Can you work these out from the model? Positions are in its coordinate system, mm. Face numbers are marked on the shaded views. A direction names the side the tool comes from. Give positions to 0.01 mm unless a question says otherwise; leave off trailing zeros. Loops run counter-clockwise (first coordinate to the right, second up) from the corner with the lowest first, then second, coordinate; pieces in that order, holes last. Notation, with made-up numbers: M -7,36.25 L 47,36.25 A34 cw 47,70.25 Z; hole C -37.5,82.25 d7. An arc over 180 degrees is marked long. One line per item, written item: value. Start each with the question number.
from build123d import *

# Parameters (mm, degrees)
BOSS_EXTRUDE2_DEPTH  = 15
BOSS_EXTRUDE3_DEPTH  = 5
SKETCH7_R            = 3.75
BOSS_EXTRUDE9_DEPTH  = 10
SKETCH9_R            = 1.375
CUT_EXTRUDE5_DEPTH   = 21
CUT_EXTRUDE9_REACH   = 131.287
SKETCH14_R           = 8
CUT_EXTRUDE11_REACH  = 105.053
SKETCH16_R           = 8
CUT_EXTRUDE12_REACH  = 131.287
SKETCH17_R           = 8
CUT_EXTRUDE13_REACH  = 121.393
SKETCH19_R           = 8
CUT_EXTRUDE14_REACH  = 121.393
SKETCH20_R           = 8
BOSS_EXTRUDE11_DEPTH = 55
FILLET1_R            = 10
SKETCH25_R           = 4
SKETCH25_R_2         = 1.4
BOSS_EXTRUDE12_DEPTH = 5
SKETCH24_R           = 3.75
CUT_EXTRUDE15_DEPTH  = 65
CUT_EXTRUDE17_REACH  = 105.053
SKETCH26_W           = 58.5
SKETCH26_H           = 18
BOSS_EXTRUDE13_REACH = 77
SKETCH27_R           = 4
SKETCH28_R           = 1.375
CUT_EXTRUDE18_DEPTH  = 25
SKETCH30_R           = 8
CUT_EXTRUDE19_DEPTH  = 122.75
SKETCH31_R           = 8
CUT_EXTRUDE20_DEPTH  = 1.5
SKETCH33_W           = 27
SKETCH33_H           = 4
CUT_EXTRUDE21_DEPTH  = 40
SKETCH35_R           = 1.25
SKETCH35_W           = 9
SKETCH35_H           = 9
CUT_EXTRUDE22_DEPTH  = 7.75


with BuildPart() as part:
    # Sketch1 → Boss-Extrude2 (new body)
    with BuildSketch(Plane(origin=(0, 0, 0), x_dir=(1, 0, 0), z_dir=(0, 1, 0))):
        Polygon((-43.178681761, 29.873916914), (-17.5, 45.604089113), (-17.5, 57.803420417), (17.5, 57.803420417), (17.5, 45.604089113), (43.178681761, 29.873916914), (59, 2.406681305), (59, -41.5), (-59, -41.5), (-59, 2.406681305), align=None)
        Polygon((39.481402229, 26.275231503), (12.5, 42.803420417), (12.5, 52.803420417), (-12.5, 52.803420417), (-12.5, 42.803420417), (-39.481402229, 26.275231503), (-54, 1.069636136), (-54, -38.5), (54, -38.5), (54, 1.069636136), align=None, mode=Mode.SUBTRACT)
    extrude(amount=BOSS_EXTRUDE2_DEPTH)

    # Sketch2 → Boss-Extrude3 (add)
    with BuildSketch(Plane.XZ):
        Polygon((-59, -2.406681305), (-59, 41.5), (59, 41.5), (59, -2.406681305), (43.178681761, -29.873916914), (43.178681761, -57.803420417), (-43.178681761, -57.803420417), (-43.178681761, -29.873916914), align=None)
    extrude(amount=BOSS_EXTRUDE3_DEPTH)

    # Sketch7 → Boss-Extrude9 (add)
    with BuildSketch(Plane(origin=(0, 15, 0), x_dir=(1, 0, 0), z_dir=(0, 1, 0))):
        with Locations((-59, -41.5)):
            Circle(SKETCH7_R)
        with Locations((-59, 2.406681305)):
            Circle(SKETCH7_R)
        with Locations((-43.178681761, 29.873916914)):
            Circle(SKETCH7_R)
        with Locations((-17.5, 57.803420417)):
            Circle(SKETCH7_R)
        with Locations((17.5, 57.803420417)):
            Circle(SKETCH7_R)
        with Locations((43.178681761, 29.873916914)):
            Circle(SKETCH7_R)
        with Locations((59, 2.406681305)):
            Circle(SKETCH7_R)
        with Locations((59, -41.5)):
            Circle(SKETCH7_R)
    extrude(amount=-BOSS_EXTRUDE9_DEPTH)

    # Sketch9 → Cut-Extrude5 (cut, through all)
    with BuildSketch(Plane(origin=(0, 15, 0), x_dir=(1, 0, 0), z_dir=(0, 1, 0))):
        with Locations((-59, -41.5)):
            Circle(SKETCH9_R)
        with Locations((-59, 2.406681305)):
            Circle(SKETCH9_R)
        with Locations((-17.5, 57.803420417)):
            Circle(SKETCH9_R)
        with Locations((43.178681761, 29.873916914)):
            Circle(SKETCH9_R)
        with Locations((17.5, 57.803420417)):
            Circle(SKETCH9_R)
        with Locations((-43.178681761, 29.873916914)):
            Circle(SKETCH9_R)
        with Locations((59, 2.406681305)):
            Circle(SKETCH9_R)
        with Locations((59, -41.5)):
            Circle(SKETCH9_R)
    extrude(amount=-CUT_EXTRUDE5_DEPTH, mode=Mode.SUBTRACT)

    # Sketch14 → Cut-Extrude9 (cut, up to next)
    with BuildSketch(Plane(origin=(-45.342387005, 0, -26.117529435), x_dir=(-0.499126718, 0, 0.866529006), z_dir=(-0.866529006, 0, -0.499126718)), mode=Mode.PRIVATE) as cut_extrude9_sk1:
        with Locations((11.514017709, 15)):
            Circle(SKETCH14_R)
    cut_extrude9_tool1 = extrude(cut_extrude9_sk1.sketch, amount=-CUT_EXTRUDE9_REACH, mode=Mode.PRIVATE) & part.part
    add(cut_extrude9_tool1.solids().sort_by_distance((-51.089341, 15, -16.140299))[0], mode=Mode.SUBTRACT)

    # Sketch16 → Cut-Extrude11 (cut, up to next)
    with BuildSketch(Plane(origin=(0, 0, -57.803420417), x_dir=(-1, 0, 0), z_dir=(0, 0, -1)), mode=Mode.PRIVATE) as cut_extrude11_sk1:
        with Locations((0, 15)):
            Circle(SKETCH16_R)
    cut_extrude11_tool1 = extrude(cut_extrude11_sk1.sketch, amount=-CUT_EXTRUDE11_REACH, mode=Mode.PRIVATE) & part.part
    add(cut_extrude11_tool1.solids().sort_by_distance((0, 15, -57.80342))[0], mode=Mode.SUBTRACT)

    # Sketch17 → Cut-Extrude12 (cut, up to next)
    with BuildSketch(Plane(origin=(45.342387005, 0, -26.117529435), x_dir=(-0.499126718, 0, -0.866529006), z_dir=(0.866529006, 0, -0.499126718)), mode=Mode.PRIVATE) as cut_extrude12_sk1:
        with Locations((-11.514017709, 15)):
            Circle(SKETCH17_R)
    cut_extrude12_tool1 = extrude(cut_extrude12_sk1.sketch, amount=-CUT_EXTRUDE12_REACH, mode=Mode.PRIVATE) & part.part
    add(cut_extrude12_tool1.solids().sort_by_distance((51.089341, 15, -16.140299))[0], mode=Mode.SUBTRACT)

    # Sketch19 → Cut-Extrude13 (cut, up to next)
    with BuildSketch(Plane(origin=(-25.088449392, 0, -40.955578852), x_dir=(-0.852725133, 0, 0.522359882), z_dir=(-0.522359882, 0, -0.852725133)), mode=Mode.PRIVATE) as cut_extrude13_sk1:
        with Locations((4.464611438, 15)):
            Circle(SKETCH19_R)
    cut_extrude13_tool1 = extrude(cut_extrude13_sk1.sketch, amount=-CUT_EXTRUDE13_REACH, mode=Mode.PRIVATE) & part.part
    add(cut_extrude13_tool1.solids().sort_by_distance((-28.895536, 15, -38.623445))[0], mode=Mode.SUBTRACT)

    # Sketch20 → Cut-Extrude14 (cut, up to next)
    with BuildSketch(Plane(origin=(25.088449392, 0, -40.955578852), x_dir=(-0.852725133, 0, -0.522359882), z_dir=(0.522359882, 0, -0.852725133)), mode=Mode.PRIVATE) as cut_extrude14_sk1:
        with Locations((-4.464611438, 15)):
            Circle(SKETCH20_R)
    cut_extrude14_tool1 = extrude(cut_extrude14_sk1.sketch, amount=-CUT_EXTRUDE14_REACH, mode=Mode.PRIVATE) & part.part
    add(cut_extrude14_tool1.solids().sort_by_distance((28.895536, 15, -38.623445))[0], mode=Mode.SUBTRACT)

    # Sketch21 → Boss-Extrude11 (add)
    with BuildSketch(Plane.XZ.offset(5)):
        Polygon((59, 41.5), (59, -2.406681305), (43.178681761, -29.873916914), (43.178681761, -57.803420417), (-43.178681761, -57.803420417), (-43.178681761, -29.873916914), (-59, -2.406681305), (-59, 41.5), align=None)
        Polygon((54, 38.5), (-54, 38.5), (-54, -1.069636136), (-38.178681761, -28.536871745), (-38.178681761, -52.803420417), (38.178681761, -52.803420417), (38.178681761, -28.536871745), (54, -1.069636136), align=None, mode=Mode.SUBTRACT)
    extrude(amount=BOSS_EXTRUDE11_DEPTH)

    # Fillet1
    fillet1_edges = [part.edges().sort_by_distance(p)[0] for p in [
        (43.178681761, -30, -57.803420417),
        (-43.178681761, -30, -57.803420417),
    ]]
    fillet(fillet1_edges, radius=FILLET1_R)

    # Sketch25 → Boss-Extrude12 (add)
    with BuildSketch(Plane(origin=(0, -5, 0), x_dir=(-1, 0, 0), z_dir=(0, -1, 0))):
        with Locations((-24.5, 40.5)):
            Circle(SKETCH25_R)
        with Locations((-24.5, 40.5)):
            Circle(SKETCH25_R_2, mode=Mode.SUBTRACT)
        with Locations((24.5, 40.5)):
            Circle(SKETCH25_R)
        with Locations((24.5, 40.5)):
            Circle(SKETCH25_R_2, mode=Mode.SUBTRACT)
        with Locations((24.5, -17.5)):
            Circle(SKETCH25_R)
        with Locations((24.5, -17.5)):
            Circle(SKETCH25_R_2, mode=Mode.SUBTRACT)
        with Locations((-24.5, -17.5)):
            Circle(SKETCH25_R)
        with Locations((-24.5, -17.5)):
            Circle(SKETCH25_R_2, mode=Mode.SUBTRACT)
    extrude(amount=BOSS_EXTRUDE12_DEPTH)

    # Sketch24 → Cut-Extrude15 (cut)
    with BuildSketch(Plane.XZ.offset(60)):
        with Locations((59, 41.5)):
            Circle(SKETCH24_R)
        with Locations((59, -2.406681305)):
            Circle(SKETCH24_R)
        with Locations((43.178681761, -29.873916914)):
            Circle(SKETCH24_R)
        with Locations((17.5, -57.803420417)):
            Circle(SKETCH24_R)
        with Locations((-17.5, -57.803420417)):
            Circle(SKETCH24_R)
        with Locations((-43.178681761, -29.873916914)):
            Circle(SKETCH24_R)
        with Locations((-59, -2.406681305)):
            Circle(SKETCH24_R)
        with Locations((-59, 41.5)):
            Circle(SKETCH24_R)
    extrude(amount=-CUT_EXTRUDE15_DEPTH, mode=Mode.SUBTRACT)

    # Sketch26 → Cut-Extrude17 (cut, up to next)
    with BuildSketch(Plane.XY.offset(41.5), mode=Mode.PRIVATE) as cut_extrude17_sk1:
        with Locations((0, -19)):
            Rectangle(SKETCH26_W, SKETCH26_H)
    cut_extrude17_tool1 = extrude(cut_extrude17_sk1.sketch, amount=-CUT_EXTRUDE17_REACH, mode=Mode.PRIVATE) & part.part
    add(cut_extrude17_tool1.solids().sort_by_distance((0, -19, 41.5))[0], mode=Mode.SUBTRACT)

    # Sketch27 → Boss-Extrude13 (add, up to next)
    with BuildSketch(Plane(origin=(0, -60, 0), x_dir=(-1, 0, 0), z_dir=(0, -1, 0)), mode=Mode.PRIVATE) as boss_extrude13_sk1:
        with Locations((-51.25, -35.75)):
            Circle(SKETCH27_R)
    boss_extrude13_tool1 = extrude(boss_extrude13_sk1.sketch, amount=-BOSS_EXTRUDE13_REACH, mode=Mode.PRIVATE) - part.part
    add(boss_extrude13_tool1.solids().sort_by_distance((51.25, -60, 35.75))[0])
    # Sketch27 → Boss-Extrude13 (add, up to next)
    with BuildSketch(Plane(origin=(0, -60, 0), x_dir=(-1, 0, 0), z_dir=(0, -1, 0)), mode=Mode.PRIVATE) as boss_extrude13_sk2:
        with Locations((-35.428681761, 50.053420417)):
            Circle(SKETCH27_R)
    boss_extrude13_tool2 = extrude(boss_extrude13_sk2.sketch, amount=-BOSS_EXTRUDE13_REACH, mode=Mode.PRIVATE) - part.part
    add(boss_extrude13_tool2.solids().sort_by_distance((35.428682, -60, -50.05342))[0])
    # Sketch27 → Boss-Extrude13 (add, up to next)
    with BuildSketch(Plane(origin=(0, -60, 0), x_dir=(-1, 0, 0), z_dir=(0, -1, 0)), mode=Mode.PRIVATE) as boss_extrude13_sk3:
        with Locations((35.428681761, 50.053420417)):
            Circle(SKETCH27_R)
    boss_extrude13_tool3 = extrude(boss_extrude13_sk3.sketch, amount=-BOSS_EXTRUDE13_REACH, mode=Mode.PRIVATE) - part.part
    add(boss_extrude13_tool3.solids().sort_by_distance((-35.428682, -60, -50.05342))[0])
    # Sketch27 → Boss-Extrude13 (add, up to next)
    with BuildSketch(Plane(origin=(0, -60, 0), x_dir=(-1, 0, 0), z_dir=(0, -1, 0)), mode=Mode.PRIVATE) as boss_extrude13_sk4:
        with Locations((51.25, -35.75)):
            Circle(SKETCH27_R)
    boss_extrude13_tool4 = extrude(boss_extrude13_sk4.sketch, amount=-BOSS_EXTRUDE13_REACH, mode=Mode.PRIVATE) - part.part
    add(boss_extrude13_tool4.solids().sort_by_distance((-51.25, -60, 35.75))[0])

    # Sketch28 → Cut-Extrude18 (cut)
    with BuildSketch(Plane(origin=(0, -60, 0), x_dir=(-1, 0, 0), z_dir=(0, -1, 0))):
        with Locations((-51.25, -35.75)):
            Circle(SKETCH28_R)
        with Locations((-35.428681761, 50.053420417)):
            Circle(SKETCH28_R)
        with Locations((35.428681761, 50.053420417)):
            Circle(SKETCH28_R)
        with Locations((51.25, -35.75)):
            Circle(SKETCH28_R)
    extrude(amount=-CUT_EXTRUDE18_DEPTH, mode=Mode.SUBTRACT)

    # Sketch30 → Cut-Extrude19 (cut, through all)
    with BuildSketch(Plane.ZY.offset(59)):
        with Locations((13.34, 15)):
            Circle(SKETCH30_R)
    extrude(amount=-CUT_EXTRUDE19_DEPTH, mode=Mode.SUBTRACT)

    # Sketch31 → Cut-Extrude20 (cut)
    with BuildSketch(Plane(origin=(0, 0, 38.5), x_dir=(-1, 0, 0), z_dir=(0, 0, -1))):
        with Locations((-38, 15)):
            Circle(SKETCH31_R)
    extrude(amount=-CUT_EXTRUDE20_DEPTH, mode=Mode.SUBTRACT)

    # Sketch33 → Cut-Extrude21 (cut)
    with BuildSketch(Plane.XZ.offset(60)):
        with Locations((0, -52.803420417)):
            Rectangle(SKETCH33_W, SKETCH33_H)
    extrude(amount=-CUT_EXTRUDE21_DEPTH, mode=Mode.SUBTRACT)

    # Sketch35 → Cut-Extrude22 (cut, through all)
    with BuildSketch(Plane.XY.offset(-54.803420417)):
        with Locations((10.5, -35.5)):
            Circle(SKETCH35_R)
        with Locations((-10.5, -35.5)):
            Circle(SKETCH35_R)
        with Locations((-10.5, -23)):
            Circle(SKETCH35_R)
        with Locations((10.5, -23)):
            Circle(SKETCH35_R)
        with Locations((0, -35.5)):
            Rectangle(SKETCH35_W, SKETCH35_H)
    extrude(amount=-CUT_EXTRUDE22_DEPTH, mode=Mode.SUBTRACT)


solid = part.part
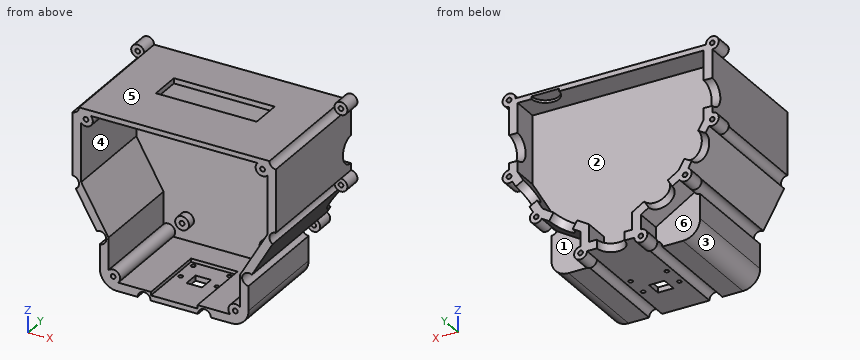
Q1. If we mould it in two halves opening along X, with no side actions, what happens to the marked faces 1, 2 and 3? For each: released by +X, released by -X, zero draft, split by the parting line, or undercut.
Q2. For P1, Ø1.5, axis at y = -33.5, z = -56, coming from the +X side; P2, Ø12, axis at x = 29.5, z = -2.5, coming from the +Y side; P3, Ø14, axis at x = 5, y = -22.5, coming from the -Z side; P4, Ø3, axis at x = -51.25, z = 35.75, coming from the -Y side, each with a flat end and sliding along its axis, tell me the tip position at first contact or that it passes through.
Q3. If we section it at A-A, the plane x = -2: Write out the boundary of the cut face in (y, z), plus the area to 3 significant figures.
Q4. If we section it at B-B, the plane y = -52.5: Give the number of separate pieces and of enclosed holes in the cut face, plus the area to 3 significant figures.
Q5. I need wall thicknesses on line 1 along Y through (x, z) = (10.5, -55.5); line 2 along Z through (x, y) = (-24.5, -7.65); line 3 along X through (y, z) = (-43, 35.75) (3 decimals). Which ranges of each line are inside material? Lowest first, please.
Q6. Which directions (+Z, -Z, +X, -X, +Y, -Y) give clear straight access to the entire face, cutting with the end or side of a thin tool? Please do the marked faces 4, 5 and 6.
Response:
1. face 1: zero draft
1. face 2: undercut
1. face 3: released by -X
2. P1: x = 39.85
2. P2: y = 0
2. P3: z = -57.8
2. P4: y = -60
3. outline: M -60,-57.8 L -40,-57.8 L -40,-54.8 L -60,-54.8 Z; M -60,38.5 L -28,38.5 L -28,41.5 L -60,41.5 Z; M -31,-57.8 L 7.25,-57.8 L 7.25,-52.8 L 0,-52.8 L 0,38.5 L 15,38.5 L 15,41.5 L -10,41.5 L -10,38.5 L -5,38.5 L -5,-52.8 L -20,-52.8 L -20,-54.8 L -31,-54.8 Z
3. area: 857 mm^2
4. separate pieces: 1
4. enclosed holes: 5
4. area: 1,630 mm^2
5. line 1: -60 to -36.75, -34.25 to -24.25, -21.75 to 15
5. line 2: -57.8 to -52.8, -44.5 to -41.9, -39.1 to -36.5, 13.5 to 16.1, 18.9 to 21.5, 38.5 to 41.5
5. line 3: -59 to -52.625, -49.875 to -47.25, 47.25 to 49.875, 52.625 to 59
6. face 4: -Y
6. face 5: +Z, +Y, -Y
6. face 6: -Z, -X, +Y
